Geometry check sheet. Reference: the model listing, model coordinates, mm. A direction names the side the tool comes from. Give positions to 0.01 mm unless a question says otherwise; leave off trailing zeros. Loops run counter-clockwise (first coordinate to the right, second up) from the corner with the lowest first, then second, coordinate; pieces in that order, holes last. Notation, with made-up numbers: (62, 67) - (101, 67) arc R20 ccw to (101, 81) - close; hole circle Ø8 at (-9.75, 20.5). An arc over 180 degrees is marked (long way). Write item = value, one per line. Start each with the question number.
from build123d import *

# Parameters (mm, degrees)
EXTRUDE_1_DEPTH        = 63.5
SKETCH_2_R             = 2
EXTRUDE_4_DEPTH        = 0.5
PATTERN_LINEAR_2_COUNT = 9
PATTERN_LINEAR_2_PITCH = 7.4
SKETCH_4_R             = 1.6
CUT_EXTRUDE_1_DEPTH    = 10.5
PATTERN_LINEAR_3_COUNT = 3
PATTERN_LINEAR_3_PITCH = 15
CUT_EXTRUDE_2_DEPTH    = 20
FILLET_1_R             = 6
FILLET_2_R             = 4


with BuildPart() as part:
    # 草图1 → 凸台-拉伸1 (new body)
    with BuildSketch(Plane.XY):
        Polygon((12.374107166, 7.245427509), (12.727660556, 7.5989809), (10.663320728, 9.663320728), (8, 7), (0, 7), (0, 2.871320344), (8, 2.871320344), (10.252786822, 5.124107166), align=None)
    extrude(amount=EXTRUDE_1_DEPTH)

    # 草图2 → 凸台-拉伸4 (add)
    with BuildSketch(Plane(origin=(2.564339828, -2.564339828, 0), x_dir=(0, 0, -1), z_dir=(0.7071067811865562, -0.7071067811865389, 0))):
        with Locations(Location((-2, 12.373106012, 0), (0, 0, 90))):
            Circle(SKETCH_2_R)
    extrude_4 = extrude(amount=EXTRUDE_4_DEPTH)

    # 阵列(线性)2: 凸台-拉伸4 ×9
    with Locations(*[(0, 0, i * PATTERN_LINEAR_2_PITCH) for i in range(1, PATTERN_LINEAR_2_COUNT)]):
        add(extrude_4)

    # 草图4 → 切除-拉伸1 (cut)
    with BuildSketch(Plane(origin=(0, 7, 0), x_dir=(1, 0, 0), z_dir=(0, 1, 0))):
        with Locations(Location((4, -4, 0), (0, 0, 180))):
            Circle(SKETCH_4_R)
    cut_extrude_1 = extrude(amount=-CUT_EXTRUDE_1_DEPTH, mode=Mode.SUBTRACT)

    # 阵列(线性)3: 切除-拉伸1 ×3
    with Locations(*[(0, 0, i * PATTERN_LINEAR_3_PITCH) for i in range(1, PATTERN_LINEAR_3_COUNT)]):
        add(cut_extrude_1, mode=Mode.SUBTRACT)

    # 草图5 → 切除-拉伸2 (cut, symmetric)
    with BuildSketch(Plane(origin=(0, 7, 0), x_dir=(1, 0, 0), z_dir=(0, 1, 0))):
        with BuildLine():
            Line((4, -40.973787182), (0.723391823, -36.294305745))
            ThreePointArc((0.723391823, -36.294305745), (0.185132197, -35.202823198), (0, -34))
            Line((0, -34), (-5.450044849, -34))
            Line((-5.450044849, -34), (-5.450044849, -68.07872052))
            Line((-5.450044849, -68.07872052), (16.294093075, -68.07872052))
            Line((16.294093075, -68.07872052), (16.294093075, -55.8))
            Line((16.294093075, -55.8), (4, -55.8))
            Line((4, -55.8), (4, -40.973787182))
        make_face()
    extrude(amount=CUT_EXTRUDE_2_DEPTH, both=True, mode=Mode.SUBTRACT)

    # 圆角1
    fillet_1_edges = [part.edges().sort_by_distance(p)[0] for p in [
        (4, 4.935660172, 55.8),
    ]]
    fillet(fillet_1_edges, radius=FILLET_1_R)

    # 圆角2
    fillet_2_edges = [part.edges().sort_by_distance(p)[0] for p in [
        (4, 4.935660172, 40.973787182),
    ]]
    fillet(fillet_2_edges, radius=FILLET_2_R)


solid = part.part
1) Release check for a two-part mould opening along Y. For faces 1 (the face through (4, 7, 21)), 2 (the face through (3.82, 4.91, 41.05)), 3 (the face through (11.18, 5.7, 29.65)) record: pulls with the +Y half, pulls with the -Y half, needs draft (parallel to the pull), parting line crosses it, or undercut.
2) Gauge pin test, flat ends, axial feed: P1, Ø1, axis at y = 9, z = 11, coming from the +X side; P2, Ø1.9, axis at x = 4, z = 34, coming from the -Y side; P3, Ø4, axis at x = 4, z = 4, coming from the +Y side; P4, Ø1, axis at x = 2, y = 5, coming from the +Z side. Record the tip position at first contact, or that the pin passes through.
3) Tool access check on faces 4 (the face through (4, 5, 46)), 5 (the face through (11.18, 5.7, 7.45)). Record the directions out of +Z, -Z, +X, -X, +Y, -Y that give a thin tool (end or side, any length) a straight path to the whole face; none if there is none.
4) Cross-section at A-A on x = 4.75. Enter the section's corners in (y, z).
5) Cross-section at B-B on y = 8.5. Enter the section's corners in (x, z), and give its area (3 significant figures).
6) Material ranges on line 1 along Z through (x, y) = (4.5, 3.5); line 2 along Z through (x, y) = (4.75, 4.75); line 3 along Y through (x, z) = (7.75, 27), recorded low to high.
Checked values:
q1.face_1 = pulls with the +Y half
q1.face_2 = needs draft
q1.face_3 = undercut
q2.P1 = 11.83
q2.P2 = through
q2.P3 = 7
q2.P4 = 38.83
q3.face_4 = +Z, -X, +Y, -Y
q3.face_5 = none
q4.outline = (2.87, 0) - (7, 0) - (7, 2.59) - (2.87, 2.59) - close; (2.87, 5.41) - (7, 5.41) - (7, 17.59) - (2.87, 17.59) - close; (2.87, 20.41) - (7, 20.41) - (7, 32.59) - (2.87, 32.59) - close; (2.87, 35.41) - (7, 35.41) - (7, 52.7) - (2.87, 52.7) - close
q5.outline = (9.5, 0) - (11.83, 0) - (11.83, 55.8) - (10, 55.8) arc R6 ccw to (9.5, 55.78) - close
q5.area = 130 mm²
q6.line_1 = 0 to 2.48, 5.52 to 17.48, 20.52 to 32.48, 35.52 to 52.2
q6.line_2 = 0 to 2.59, 5.41 to 17.59, 20.41 to 32.59, 35.41 to 52.7
q6.line_3 = 2.87 to 7
